Input: part model. Units: mm. Frame: model coordinates. Face numbers are marked on the shaded views. A direction names the side the tool comes from. Coordinates: 2 decimals unless noted, no trailing zeros. Loops run counter-clockwise (first coordinate to the right, second up) from the corner with the lowest first, then second, coordinate; pieces in that order, holes last.
(1) Section C-C, the plane x = 8. Return loops of the section in (y, z).
(2) Contact query for flat-ended pins moving along their axis: P1, Ø7, axis at x = 0, z = 7, coming from the -Y side; P2, Ø10, axis at x = -13.5, y = 10.5, coming from the -Z side; P3, Ø21.5, axis at x = 6, z = -0.5, coming from the -Y side; P4, Ø6, axis at x = 6.5, y = 8, coming from the +Z side. Output: stop coordinate, or through.
(3) Set-up query: the marked faces 4, 5, 6 and 7. Return all of +Z, -Z, +X, -X, +Y, -Y with unobstructed straight access to the full face (end or side cutting, diameter ignored); none if empty.
(4) Mould query, pull axis X, two halves, no side actions, for the marked faces 1, 2 and 3. Classes: released by +X, released by -X, zero draft, split by the parting line, or undercut.
(5) Line query: L1, parallel to X at y = 10, z = 18; L2, parallel to Z at x = -20, y = 10; L3, parallel to Y at x = 20, z = 10. Output: solid intervals per line, ascending.
(6) Section A-A, the plane y = 10. Give the number of separate pieces and of enclosed holes in the cut face, then the cut area to 3 significant figures.
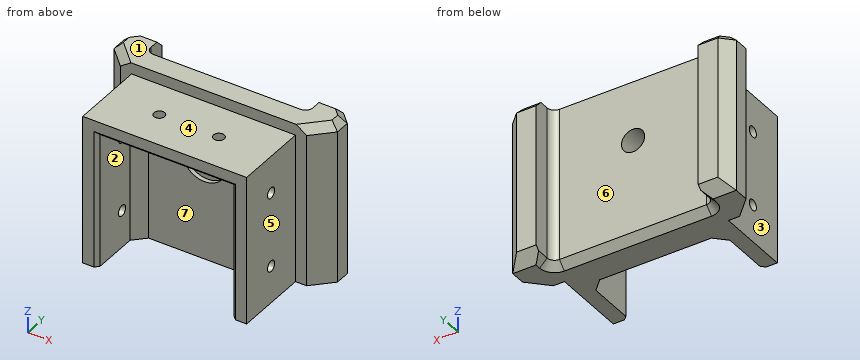
Autodesk Inventor part; units mm, degrees
ref_plane "YZ Plane" through (0, 0, 0) normal (1, 0, 0) x (0, 1, 0)
ref_plane "XZ Plane" through (0, 0, 0) normal (0, 1, 0) x (-1, 0, 0)
ref_plane "XY Plane" through (0, 0, 0) normal (0, 0, 1) x (1, 0, 0)
sketch "Sketch1" plane through (0, 0, 0) normal (0, 1, 0) x (-1, 0, 0)
  line L0 (22, 20) -> (-22, 20)
  line L1 (-22, 20) -> (-22, -20)
  line L2 (-22, -20) -> (22, -20)
  line L3 (22, -20) -> (22, 20)
  line L4 (0, -20) -> (0, 20)
  line L5 (22, 0) -> (-22, 0)
  point P0 (0, 0)
  dimension "d0" = 44
  dimension "d1" = 40
extrude "Extrusion1" add sketch "Sketch1" along normal blind 20
sketch "Sketch2" plane through (0, 20, 0) normal (0, 1, 0) x (1, 0, 0)
  line L0 (22, 20) -> (-22, 20)
  line L1 (-22, 20) -> (-22, -20)
  line L2 (-22, -20) -> (22, -20)
  line L3 (22, -20) -> (22, 20)
  line L4 (-30, -41.7016) -> (-30, 48.9081)
  line L5 (30, 51.5024) -> (30, -37.5698)
  line L6 (-22, -20) -> (22, -20)
  line L7 (-22, -20) -> (-30, -20)
  line L8 (-22, 20) -> (-22, -20)
  line L9 (-22, 20) -> (-30, 20)
  line L10 (22, -20) -> (22, 20)
  line L11 (22, 20) -> (30, 20)
  line L12 (22, -20) -> (30, -20)
  point P0 (0, 0)
  dimension "d4" = 30
  dimension "d5" = 30
extrude "Extrusion2" add sketch "Sketch2" along normal blind 12
sketch "Sketch3" plane through (0, 32, 0) normal (0, 1, 0) x (1, 0, 0)
  line L0 (22, 20) -> (-22, 20)
  line L1 (-22, -20) -> (22, -20)
  line L2 (-21.75, 20) -> (21.75, 20)
  line L3 (21.75, 20) -> (21.75, -20)
  line L4 (21.75, -20) -> (-21.75, -20)
  line L5 (-21.75, -20) -> (-21.75, 20)
  line L6 (-21.75, 0) -> (21.75, 0)
  point P0 (0, 0)
  dimension "d8" = 21.75
  dimension "d9" = 21.75
extrude "Extrusion3" cut sketch "Sketch3" against normal blind 6.5
fillet "Fillet1" radius 2 2 edges at (-21.75, 25.5, 0) (21.75, 25.5, 0)
sketch "Sketch4" plane through (-22, 0, 20) normal (0, 0, 1) x (1, 0, 0)
  line L0 (0.25, 27.5) -> (0.25, 32)
  line L1 (-8, 32) -> (0.25, 32)
  line L2 (-8, 20) -> (-8, 32)
  line L3 (-8, 20) -> (0, 20)
  line L4 (0, 0) -> (0, 20)
  line L5 (0, 0) -> (44, 0)
  line L6 (44, 0) -> (44, 20)
  line L7 (44, 20) -> (52, 20)
  line L8 (52, 20) -> (52, 32)
  line L9 (43.75, 32) -> (52, 32)
  line L10 (43.75, 32) -> (43.75, 27.5)
  arc A0 (41.75, 25.5) -> (43.75, 27.5) centre (41.75, 27.5) ccw
  line L11 (41.75, 25.5) -> (2.25, 25.5)
  arc A1 (0.25, 27.5) -> (2.25, 25.5) centre (2.25, 27.5) ccw
  line L12 (-8, 20) -> (0, 20)
  line L13 (0, 20) -> (44, 20)
  point P0 (22, 0)
extrude "Extrusion4" add sketch "Sketch4" along normal blind 3 contours A1 L11 A0 L10 L9 L8 L7 L13 L3 L2 L1 L0
chamfer "Chamfer1" distance 3 angle 45 4 edges at (25.875, 32, -20) (-25.875, 32, -20) (30, 32, 1.5) (-30, 32, 1.5)
sketch "Sketch5" plane through (22, 0, -20) normal (0, 0, -1) x (-1, 0, 0)
  line L0 (0, 0) -> (44, 0)
  line L1 (4, 0) -> (40, 0)
  line L2 (40, 0) -> (40, 16.2778)
  line L3 (40, 16.2778) -> (4, 16.2778)
  line L4 (4, 16.2778) -> (4, 0)
  line L5 (0, 0) -> (0, 20)
  line L6 (44, 0) -> (44, 20)
  point P0 (22, 0)
  dimension "d18" = 4
  dimension "d19" = 4
extrude "Extrusion5" cut sketch "Sketch5" against normal blind 36
chamfer "Chamfer2" distance 3 angle 45 3 edges at (18, 16.2778, -2) (-18, 16.2778, -2) (0, 16.2778, 16)
sketch "Sketch6" plane through (-22, 0, -20) normal (-1, 0, 0) x (0, 0, 1)
  line L0 (10, 10) -> (30, 10) construction
  line L1 (0, 0) -> (0, 20)
  line L2 (0, 20) -> (43, 20)
  point P0 (20, 0)
  dimension "d25" = 10
  dimension "d26" = 10
  dimension "d53" = 20
hole "Hole1" at (-22, 10, -10) at (-22, 10, 10) direction (1, 0, 0) diameter 2.9 end through all
sketch "Sketch7" plane through (-22, 0, 20) normal (0, 0, 1) x (1, 0, 0)
  line L0 (14, 10) -> (30, 10) construction
  line L1 (-8, 20) -> (52, 20)
  line L2 (0, 0) -> (0, 20)
  point P0 (22, 0)
  dimension "d34" = 10
  dimension "d35" = 16
  dimension "d36" = 14
hole "Hole2" at (-8, 10, 20) at (8, 10, 20) direction (0, 0, -1) diameter 2.9 end through all
chamfer "Chamfer3" distance 1 angle 45 3 edges at (18, 0, -2) (0, 0, 16) (-18, 0, -2)
chamfer "Chamfer4" distance 2 angle 45 5 edges at (0, 25.5, -20) (21.1642, 26.0858, -20) (21.75, 28.25, -20) (-21.1642, 26.0858, -20) (-21.75, 28.25, -20)
chamfer "Chamfer5" distance 5 angle 45 2 edges at (30, 20, 1.5) (-30, 20, 1.5)
chamfer "Chamfer6" distance 2 angle 45 8 edges at (-27.5, 22.5, 23) (-30, 27, 23) (-28.5, 30.5, 23) (-24.375, 32, 23) (27.5, 22.5, 23) (30, 27, 23) (28.5, 30.5, 23) (24.375, 32, 23)
sketch "Sketch8" plane through (0, 25.5, 0) normal (0, 1, 0) x (1, 0, 0)
  line L0 (19.75, 20) -> (-19.75, 20)
  point P0 (0, 0)
  point P1 (0, -7)
  dimension "d57" = 27
hole "Hole3" at (0, 25.5, 7) direction (0, -1, 0) diameter 6.2 end through all
sketch "Sketch9" plane through (-15, 16.2778, -20) normal (0, -1, 0) x (1, 0, 0)
  circle A0 centre (15, 27) radius 3.1
  circle A1 centre (15, 27) radius 5.9
  point P0 (15, 20)
  dimension "d65" = 2.8
extrude "Extrusion6" cut sketch "Sketch9" against normal blind 1.2
properties part number "Camera mount"
Report:
1. outline: (0, 17) - (1, 16) - (8.55, 16) - (8.55, 20) - (0, 20) - close; (11.45, 16) - (13.28, 16) - (16.28, 13) - (16.28, -20) - (23.5, -20) - (25.5, -18) - (25.5, 23) - (20, 23) - (20, 20) - (11.45, 20) - close
2. P1: stops at y = 17.48
2. P2: stops at z = -20
2. P3: stops at y = 14.53
2. P4: stops at z = 20
3. face 4: +Z, +X, -X, -Y
3. face 5: +Z, -Z, +X, -Y
3. face 6: +Z, -Z, +Y
3. face 7: -Z, -Y
4. face 1: zero draft
4. face 2: undercut
4. face 3: released by -X
5. L1: x = -22 to -9.45, -6.55 to 6.55, 9.45 to 22
5. L2: z = -20 to -11.45, -8.55 to 8.55, 11.45 to 20
5. L3: y = 0 to 8.55, 11.45 to 25.52
6. separate pieces: 7
6. enclosed holes: 0
6. area: 394 mm2
